```python
from build123d import *

# Parameters (mm, degrees)
F1_DEPTH      = 300
F1_DEPTH_BACK = 300


with BuildPart() as f1:
    # F0 (on Right) → F1 (new body, two sides)
    with BuildSketch(Plane.YZ) as f1_sk:
        with BuildLine():
            Line((110.183008, 157.357644), (5.9717, 8.528471))
            ThreePointArc((5.9717, 8.528471), (-1.176369, 2.259783), (-10.411341, 0))
            Line((-10.411341, 0), (-36.606026, 0))
            Line((-36.606026, 0), (-36.590081, -4))
            Line((-36.590081, -4), (-10.411341, -4))
            ThreePointArc((-10.411341, -4), (0.670626, -1.28826), (9.248308, 6.234166))
            Line((9.248308, 6.234166), (113.459616, 155.063338))
            ThreePointArc((113.459616, 155.063338), (147.770346, 185.15304), (192.098213, 196))
            Line((192.098213, 196), (231.673377, 196))
            ThreePointArc((231.673377, 196), (242.48282, 191.796437), (247.612492, 181.394492))
            Line((247.612492, 181.394492), (261.915687, 17.908216))
            ThreePointArc((261.915687, 17.908216), (269.610202, 2.305292), (285.824377, -4.000046))
            Line((285.824377, -4.000046), (339.588671, -4.000007))
            ThreePointArc((339.588671, -4.000007), (350.670628, -1.288263), (359.248303, 6.234158))
            Line((359.248303, 6.234158), (463.459616, 155.063338))
            ThreePointArc((463.459616, 155.063338), (497.770346, 185.15304), (542.098213, 196))
            Line((542.098213, 196), (581.673377, 196))
            ThreePointArc((581.673377, 196), (591.80723, 192.05916), (596.616297, 182.307336))
            Line((596.616297, 182.307336), (610.919489, 18.821106))
            ThreePointArc((610.919489, 18.821106), (618.613997, 3.218188), (634.828161, -3.087156))
            Line((634.828161, -3.087156), (688.592464, -3.087156))
            ThreePointArc((688.592464, -3.087156), (699.674431, -0.375416), (708.252113, 7.14701))
            Line((708.252113, 7.14701), (812.463422, 155.976182))
            ThreePointArc((812.463422, 155.976182), (846.774151, 186.065884), (891.102018, 196.912844))
            Line((891.102018, 196.912844), (930.677182, 196.912844))
            ThreePointArc((930.677182, 196.912844), (940.811035, 192.972004), (945.620102, 183.22018))
            Line((945.620102, 183.22018), (959.923294, 19.733951))
            ThreePointArc((959.923294, 19.733951), (967.617802, 4.131032), (983.831967, -2.174311))
            Line((983.831967, -2.174311), (1037.59627, -2.174311))
            ThreePointArc((1037.59627, -2.174311), (1048.678236, 0.537429), (1057.255919, 8.059854))
            Line((1057.255919, 8.059854), (1161.467227, 156.889026))
            ThreePointArc((1161.467227, 156.889026), (1195.777956, 186.978728), (1240.105823, 197.825689))
            Line((1240.105823, 197.825689), (1279.680987, 197.825689))
            ThreePointArc((1279.680987, 197.825689), (1289.81484, 193.884849), (1294.623908, 184.133025))
            Line((1294.623908, 184.133025), (1308.927099, 20.646795))
            ThreePointArc((1308.927099, 20.646795), (1316.621607, 5.043877), (1332.835772, -1.261467))
            Line((1332.835772, -1.261467), (1386.600075, -1.261467))
            ThreePointArc((1386.600075, -1.261467), (1397.682042, 1.450273), (1406.259724, 8.972698))
            Line((1406.259724, 8.972698), (1510.471032, 157.801871))
            ThreePointArc((1510.471032, 157.801871), (1544.781762, 187.891573), (1589.109629, 198.738533))
            Line((1589.109629, 198.738533), (1628.684792, 198.738533))
            ThreePointArc((1628.684792, 198.738533), (1638.818646, 194.797693), (1643.627713, 185.045869))
            Line((1643.627713, 185.045869), (1659.528175, 3.302754))
            Line((1659.528175, 3.302754), (1663.393974, 3.302754))
            Line((1663.393974, 3.302754), (1663.393974, 5.01132))
            Line((1663.393974, 5.01132), (1647.612492, 185.394492))
            ThreePointArc((1647.612492, 185.394492), (1641.521006, 197.746802), (1628.684792, 202.738533))
            Line((1628.684792, 202.738533), (1589.109629, 202.738533))
            ThreePointArc((1589.109629, 202.738533), (1542.934767, 191.439616), (1507.194424, 160.096176))
            Line((1507.194424, 160.096176), (1402.983116, 11.267004))
            ThreePointArc((1402.983116, 11.267004), (1395.835047, 4.998316), (1386.600075, 2.738533))
            Line((1386.600075, 2.738533), (1332.835772, 2.738533))
            ThreePointArc((1332.835772, 2.738533), (1319.323968, 7.992986), (1312.911878, 20.995418))
            Line((1312.911878, 20.995418), (1298.608686, 184.481648))
            ThreePointArc((1298.608686, 184.481648), (1292.517201, 196.833958), (1279.680987, 201.825689))
            Line((1279.680987, 201.825689), (1240.105823, 201.825689))
            ThreePointArc((1240.105823, 201.825689), (1193.930962, 190.526772), (1158.190619, 159.183332))
            Line((1158.190619, 159.183332), (1053.97931, 10.35416))
            ThreePointArc((1053.97931, 10.35416), (1046.831242, 4.085472), (1037.59627, 1.825689))
            Line((1037.59627, 1.825689), (983.831967, 1.825689))
            ThreePointArc((983.831967, 1.825689), (970.320163, 7.080142), (963.908073, 20.082574))
            Line((963.908073, 20.082574), (949.604881, 183.568803))
            ThreePointArc((949.604881, 183.568803), (943.513396, 195.921114), (930.677182, 200.912844))
            Line((930.677182, 200.912844), (891.102018, 200.912844))
            ThreePointArc((891.102018, 200.912844), (844.927157, 189.613928), (809.186814, 158.270488))
            Line((809.186814, 158.270488), (704.975505, 9.441316))
            ThreePointArc((704.975505, 9.441316), (697.827437, 3.172628), (688.592464, 0.912844))
            Line((688.592464, 0.912844), (634.828161, 0.912844))
            ThreePointArc((634.828161, 0.912844), (621.316357, 6.167298), (614.904268, 19.169729))
            Line((614.904268, 19.169729), (600.601076, 182.655959))
            ThreePointArc((600.601076, 182.655959), (594.50959, 195.008269), (581.673377, 200))
            Line((581.673377, 200), (542.098213, 200))
            ThreePointArc((542.098213, 200), (495.923351, 188.701083), (460.183008, 157.357644))
            Line((460.183008, 157.357644), (355.971695, 8.528464))
            ThreePointArc((355.971695, 8.528464), (348.823632, 2.259779), (339.588668, -7e-06))
            Line((339.588668, -7e-06), (285.824374, -4.6e-05))
            ThreePointArc((285.824374, -4.6e-05), (272.312561, 5.254403), (265.900466, 18.256839))
            Line((265.900466, 18.256839), (251.59727, 181.743115))
            ThreePointArc((251.59727, 181.743115), (245.185181, 194.745547), (231.673377, 200))
            Line((231.673377, 200), (192.098213, 200))
            ThreePointArc((192.098213, 200), (145.923351, 188.701083), (110.183008, 157.357644))
        make_face()
    extrude(amount=F1_DEPTH)
    extrude(f1_sk.sketch, amount=-F1_DEPTH_BACK)


solid = f1.part
```
The model under review builds one solid part; all positions refer to its coordinate system, in mm. A direction names the side the tool comes from. Round coordinates to 2 decimals unless told otherwise and drop trailing zeros. Write each loop counter-clockwise with the first axis right and the second up, starting at its lowest first coordinate (ties: lowest second). Pieces come first, ordered by that corner, then holes. Notation, with made-up numbers: (8.5, 27) - (66.5, 27) arc R33 cw to (66.5, 56) - close; hole circle Ø10 at (5, 37.25). An arc over 180 degrees is marked (long way). One line per question, with ' | ' between items.
Item 1: Add section A-A, the plane y = 507. Give the boundary of the cut face in (x, z), then the cut area to 3 significant figures.
Resolved:
outline: (-300, 189.35) - (300, 189.35) - (300, 193.64) - (-300, 193.64) - close | area: 2,570 mm2
Item 2: Add section C-C, the plane y = 132.5. Give the boundary of the cut face in (x, z), then the cut area to 3 significant figures.
Resolved:
outline: (-300, 175.26) - (300, 175.26) - (300, 180.3) - (-300, 180.3) - close | area: 3,020 mm2
Item 3: For faces 1 (the face through (4.2, 258.85, 98.86)), 2 (the face through (4, 911, 196.913)), list the 3-axis set-ups (+Z, -Z, +X, -X, +Y, -Y) from which the entire face can be reached by the end or side of a thin tool; tool diameter is ignored.
Resolved:
face 1: +Z, +X, -X | face 2: -Z, +X, -X
Item 4: For P1, Ø8, axis at x = 61.5, y = -26, coming from the +Z side; P2, Ø12, axis at x = -63, y = 207.5, coming from the +Z side; P3, Ø12, axis at x = -87, y = 571, coming from the -Z side, all flat-tipped, find the tip position at first contact; note any pin that passes through.
Resolved:
P1: stops at z = 0 | P2: stops at z = 200 | P3: stops at z = 196
Item 5: Add section B-B, the plane z = 91. State how many separate pieces and enclosed holes the cut face has, then the cut area to 3 significant figures.
Resolved:
separate pieces: 10 | enclosed holes: 0 | area: 26,700 mm2
Item 6: To check wall thickness, follow probe 1 along Z at (x, y) = (2, 214.5); probe 2 along Z at (x, y) = (-153.5, 339.5). State the ranges of each line that lie inside material, in increasing order.
Resolved:
probe 1: z = 196 to 200 | probe 2: z = -4 to 0
Item 7: The part is to be moulded in two halves that separate along Y. For faces 3 (the face through (4.2, 408.807, 83.985)), 4 (the face through (4, 562, 200)), 5 (the face through (4.2, 58.807, 83.985)), say which applies: pulls with the +Y half, pulls with the -Y half, needs draft (parallel to the pull), parting line crosses it, or undercut.
Resolved:
face 3: undercut | face 4: needs draft | face 5: pulls with the -Y half
